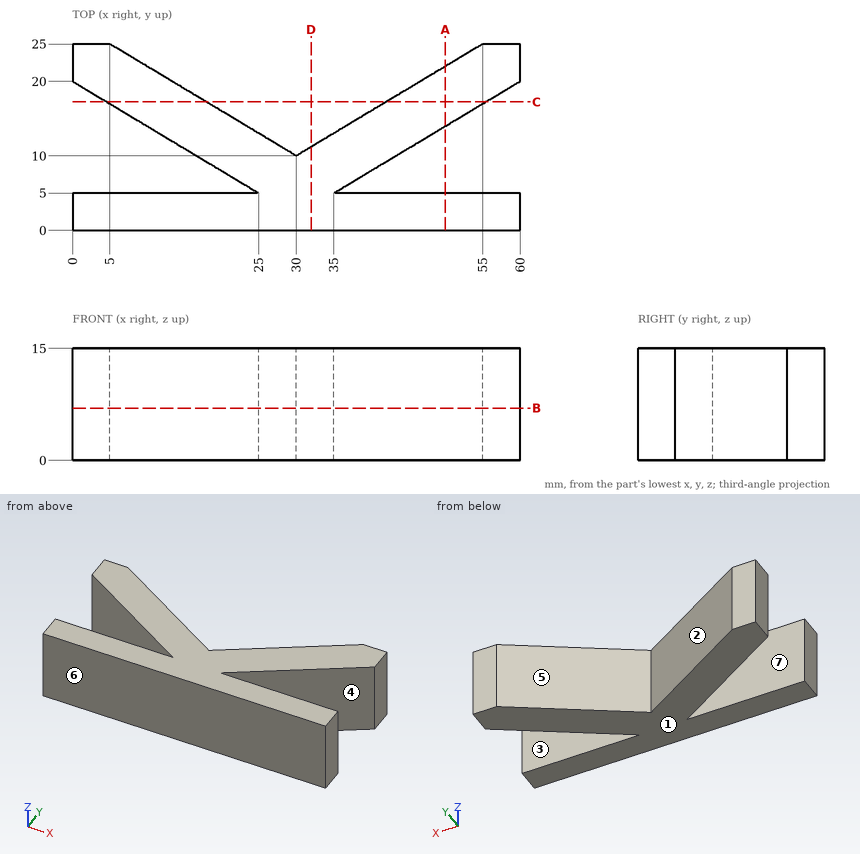
Here's the drawing with two shaded views (mm, measured from the low corner). I have some questions. A direction names the side the tool comes from. Round coordinates to 2 decimals unless told otherwise and drop trailing zeros. Loops run counter-clockwise (first coordinate to the right, second up) from the corner with the lowest first, then second, coordinate; pieces in that order, holes last.
1. Suppose I cut it at A-A, the plane x = 50. Please give me the cut outline in (y, z), and give its area (3 significant figures).
Answers:
outline: (0, 0) - (5, 0) - (5, 15) - (0, 15) - close; (14, 0) - (22, 0) - (22, 15) - (14, 15) - close
area: 195 mm2
2. For the marked faces 4, 5, 6 and 7, which set-ups out of +Z, -Z, +X, -X, +Y, -Y let a thin tool reach every point of the face, with its end or its side?
Answers:
face 4: +Z, -Z, +X
face 5: +Z, -Z, +Y
face 6: +Z, -Z, +X, -X, -Y
face 7: +Z, -Z, -X
3. Suppose I cut it at D-D, the plane x = 32. Please give me the cut outline in (y, z), and give its area (3 significant figures).
Answers:
outline: (0, 0) - (11.2, 0) - (11.2, 15) - (0, 15) - close
area: 168 mm2
4. Thinking about a two-plate mould opening in Y: for the marked faces 1, 2 and 3, which applies, released by +Y, released by -Y, zero draft, split by the parting line, or undercut?
Answers:
face 1: zero draft
face 2: released by +Y
face 3: undercut
5. If I drill on probe 1 along Y at (x, z) = (3, 8.75); probe 2 along Y at (x, z) = (44.5, 8.25); probe 3 along X at (y, z) = (15.25, 8), over which ranges is the centre line in solid material (lowest first)?
Answers:
probe 1: y = 0 to 5, 18.2 to 25
probe 2: y = 0 to 5, 10.7 to 18.7
probe 3: x = 7.92 to 21.25, 38.75 to 52.08
6. Will these pins go through, and if not, where does the flat tip stop? pin 1 (1 mm diameter, centred on y = 11.5, z = 13, fed in from +X); pin 2 (6 mm diameter, centred on y = 16, z = 13, fed in from -X); pin 3 (1.5 mm diameter, centred on x = 48.5, z = 1.5, fed in from +Y).
Answers:
pin 1: stops at x = 46.67
pin 2: stops at x = 1.67
pin 3: stops at y = 21.55
7. Suppose I cut it at C-C, the plane y = 17.25. Please give me the cut outline in (x, z).
Answers:
outline: (4.58, 0) - (17.92, 0) - (17.92, 15) - (4.58, 15) - close; (42.08, 0) - (55.42, 0) - (55.42, 15) - (42.08, 15) - close
8. Suppose I cut it at B-B, the plane z = 7. Please give me the cut outline in (x, y).
Answers:
outline: (0, 0) - (60, 0) - (60, 5) - (35, 5) - (60, 20) - (60, 25) - (55, 25) - (30, 10) - (5, 25) - (0, 25) - (0, 20) - (25, 5) - (0, 5) - close
